from build123d import *

# Parameters (mm, degrees)
F0_W      = 87
F0_H      = 86
F1_DEPTH  = 10
F2_W      = 87
F2_H      = 10
F3_DEPTH  = 76
F5_DEPTH  = 5
F7_DEPTH  = 5
F8_W      = 10
F8_H      = 19.999996
F8_H_2    = 20
F9_DEPTH  = 25
F10_W     = 10
F10_H     = 19.999996
F10_H_2   = 20
F11_DEPTH = 25


with BuildPart() as f1:
    # F0 (on Front) → F1 (new body)
    with BuildSketch(Plane.XZ):
        with Locations((43.5, 43)):
            Rectangle(F0_W, F0_H)
    extrude(amount=F1_DEPTH)

    # F2 (on face) → F3 (join)
    with BuildSketch(Plane.XZ.offset(10)):
        with Locations((43.5, 5)):
            Rectangle(F2_W, F2_H)
    extrude(amount=F3_DEPTH)

    # F4 (on face) → F5 (join)
    with BuildSketch(Plane.YZ.offset(87)):
        Polygon((-86, 15), (-86, 10), (-10, 10), (-10, 86), (-15, 86), align=None)
    extrude(amount=-F5_DEPTH)

    # F6 (on face) → F7 (join)
    with BuildSketch(Plane(origin=(0, 0, 0), x_dir=(0, -1, 0), z_dir=(-1, 0, 0))):
        Polygon((15, 86), (10, 86), (10, 10), (86, 10), (86, 15), align=None)
    extrude(amount=-F7_DEPTH)

    # F8 (on face) → F9 (cut)
    with BuildSketch(Plane.XZ.offset(10)):
        with Locations((21, 66.999998)):
            Rectangle(F8_W, F8_H)
        with Locations((21, 29)):
            Rectangle(F8_W, F8_H_2)
        with Locations((66, 66.999996)):
            Rectangle(F8_W, F8_H_2)
        with Locations((66, 29)):
            Rectangle(F8_W, F8_H_2)
    extrude(amount=-F9_DEPTH, mode=Mode.SUBTRACT)

    # F10 (on face) → F11 (cut)
    with BuildSketch(Plane.XY.offset(10)):
        with Locations((21, -29.000002)):
            Rectangle(F10_W, F10_H)
        with Locations((66, -29.000004)):
            Rectangle(F10_W, F10_H_2)
        with Locations((66, -67)):
            Rectangle(F10_W, F10_H_2)
        with Locations((21, -67)):
            Rectangle(F10_W, F10_H_2)
    extrude(amount=-F11_DEPTH, mode=Mode.SUBTRACT)


solid = f1.part
The model under review builds one solid part; all positions refer to its coordinate system, in mm. A direction names the side the tool comes from. Coordinates: 2 decimals unless noted, no trailing zeros. Order: outer loops, then holes, each group sorted by start corner. A loop starts at its lowest first (then second) coordinate and runs counter-clockwise, first axis right, second up. Notation, with made-up numbers: (-22, -8.75) -> (-10, -8.75) arc R24 cw to (-10, 19.25) -> close; hole circle Ø4 at (63, 40). An arc over 180 degrees is marked (long way). Answer in a Markdown table with one row per item.
(1) Machinability: for faces 1 (the flat face through (0, -33, 34)), 2 (the flat face through (21, -19, 5)), 3 (the flat face through (21, -5, 57)), which of the approach directions +Z, -Z, +X, -X, +Y, -Y give a long, thin tool a straight path to every point of the face, cutting with its end or side? Answer none if there is none.
Answers:
| item | result |
|---|---|
| face 1 | +Z, -Z, -X, +Y, -Y |
| face 2 | +Z, -Z |
| face 3 | +Y, -Y |
(2) Consider section D-D (y = -54.5). Write out the cut boundary in (x, z).
Answers:
| item | result |
|---|---|
| outline | (0, 0) -> (87, 0) -> (87, 46.5) -> (82, 46.5) -> (82, 10) -> (5, 10) -> (5, 46.5) -> (0, 46.5) -> close |
(3) Wall thickness on line 1 along X through (y, z) = (-25, 8); line 2 along Y through (x, z) = (17, 4); line 3 along Z through (x, y) = (65.5, -2.5): over which ranges is each line inside the solid? List them lowest first.
Answers:
| item | result |
|---|---|
| line 1 | 0 to 16, 26 to 61, 71 to 87 |
| line 2 | -86 to -77, -57 to -39, -19 to 0 |
| line 3 | 0 to 19, 39 to 57, 77 to 86 |
(4) Consider section B-B (y = -23.5). Write out the cut boundary in (x, z).
Answers:
| item | result |
|---|---|
| outline | (0, 0) -> (16, 0) -> (16, 10) -> (5, 10) -> (5, 77.5) -> (0, 77.5) -> close; (26, 0) -> (61, 0) -> (61, 10) -> (26, 10) -> close; (71, 0) -> (87, 0) -> (87, 77.5) -> (82, 77.5) -> (82, 10) -> (71, 10) -> close |
(5) Consider section C-C (x = 43). Write out the cut boundary in (y, z), plus the area to 3 significant figures.
Answers:
| item | result |
|---|---|
| outline | (-86, 0) -> (0, 0) -> (0, 86) -> (-10, 86) -> (-10, 10) -> (-86, 10) -> close |
| area | 1,620 mm² |
(6) Insertion check: pin 1 (10 mm diameter, centred on x = 56.5, y = -25.5, fed in from +Z); pin 2 (4 mm diameter, centred on x = 34, z = 70.5, fed in from +Y); pin 3 (12 mm diameter, centred on x = 23, z = 66, fed in from -Y). Each pin has a flat end and moves straight along its axis. Give the tip position at first contact, or say it passes through.
Answers:
| item | result |
|---|---|
| pin 1 | z = 10 |
| pin 2 | y = 0 |
| pin 3 | y = -10 |
(7) The part is to be moulded in two halves that separate along Z. For faces 4 (the flat face through (21, -5, 39)), 5 (the flat face through (43, -47, 10)), 6 (the flat face through (66, -5, 77)), 7 (the flat face through (26, -29, 5)), say which applies: +Z half, -Z half, draft (parallel to the pull), parting line (faces both ways), or undercut.
Answers:
| item | result |
|---|---|
| face 4 | undercut |
| face 5 | +Z half |
| face 6 | undercut |
| face 7 | draft |
(8) Consider section A-A (z = 34.5). Write out the cut boundary in (x, y), plus the area to 4 significant figures.
Answers:
| item | result |
|---|---|
| outline | (0, -66.5) -> (5, -66.5) -> (5, -10) -> (16, -10) -> (16, 0) -> (0, 0) -> close; (26, -10) -> (61, -10) -> (61, 0) -> (26, 0) -> close; (71, -10) -> (82, -10) -> (82, -66.5) -> (87, -66.5) -> (87, 0) -> (71, 0) -> close |
| area | 1,235 mm² |
